Here's how the part is built. I have some questions about the finished solid (model axes, mm). Round coordinates to 2 decimals unless told otherwise and drop trailing zeros. Order: outer loops, then holes, each group sorted by start corner. A loop starts at its lowest first (then second) coordinate and runs counter-clockwise, first axis right, second up. Notation, with made-up numbers: (30.25, 29) - (62.25, 29) arc R7 ccw to (62.25, 38) - close; hole circle Ø2 at (87.5, -28.75). An arc over 180 degrees is marked (long way). One line per item, written item: value.
from build123d import *

# Parameters (mm, degrees)
F1_DEPTH = 2.5


with BuildPart() as f1:
    # F0 (on Top) → F1 (new body)
    with BuildSketch(Plane.XY):
        Polygon((55, -55), (65, -55), (65, -52.5), (75, -52.5), (75, -45), (72.5, -45), (72.5, -35), (75, -35), (75, -25), (72.5, -25), (72.5, -15), (75, -15), (75, -5), (72.5, -5), (72.5, 5), (75, 5), (75, 15), (72.5, 15), (72.5, 25), (75, 25), (75, 35), (72.5, 35), (72.5, 45), (75, 45), (75, 52.5), (65, 52.5), (65, 55), (55, 55), (55, 52.5), (45, 52.5), (45, 55), (35, 55), (35, 52.5), (25, 52.5), (25, 55), (15, 55), (15, 52.5), (5, 52.5), (5, 55), (-5, 55), (-5, 52.5), (-15, 52.5), (-15, 55), (-25, 55), (-25, 52.5), (-35, 52.5), (-35, 55), (-45, 55), (-45, 52.5), (-55, 52.5), (-55, 55), (-65, 55), (-65, 52.5), (-75, 52.5), (-75, 45), (-72.5, 45), (-72.5, 35), (-75, 35), (-75, 25), (-72.5, 25), (-72.5, 15), (-75, 15), (-75, 5), (-72.5, 5), (-72.5, -5), (-75, -5), (-75, -15), (-72.5, -15), (-72.5, -25), (-75, -25), (-75, -35), (-72.5, -35), (-72.5, -45), (-75, -45), (-75, -52.5), (-65, -52.5), (-65, -55), (-55, -55), (-55, -52.5), (-45, -52.5), (-45, -55), (-35, -55), (-35, -52.5), (-25, -52.5), (-25, -55), (-15, -55), (-15, -52.5), (-5, -52.5), (-5, -55), (5, -55), (5, -52.5), (15, -52.5), (15, -55), (25, -55), (25, -52.5), (35, -52.5), (35, -55), (45, -55), (45, -52.5), (55, -52.5), align=None)
    extrude(amount=F1_DEPTH)


solid = f1.part
Q1. If we section it at B-B, the plane x = 51: Please give me the cut outline in (y, z).
Results list:
outline: (-52.5, 0) - (52.5, 0) - (52.5, 2.5) - (-52.5, 2.5) - close
Q2. If we section it at A-A, the plane y = 17: Please give me the cut outline in (x, z).
Results list:
outline: (-72.5, 0) - (72.5, 0) - (72.5, 2.5) - (-72.5, 2.5) - close
Q3. Will these pins go through, and if not, where does the flat tip stop? pin 1 (1.2 mm diameter, centred on y = 54, z = 1.5, fed in from +X); pin 2 (0.8 mm diameter, centred on y = -19.5, z = 0.5, fed in from +X); pin 3 (0.8 mm diameter, centred on x = 73.5, z = 1.5, fed in from +Y).
Results list:
pin 1: x = 65
pin 2: x = 72.5
pin 3: y = 52.5
Q4. If I drill on line 1 along X through (y, z) = (40.5, 0.95); line 2 along Y through (x, z) = (12.5, 0.2), over which ranges is the centre line in solid material (lowest first)?
Results list:
line 1: -72.5 to 72.5
line 2: -52.5 to 52.5
